```python
from build123d import *

# Parameters (mm, degrees)
F2_DEPTH = 3.2
F3_DEPTH = 3.15


with BuildPart() as f2:
    # F1 (on Front) → F2 (new body, symmetric)
    with BuildSketch(Plane.XZ):
        with BuildLine():
            Line((12, 6.3), (12, 0))
            Line((12, 0), (-12, 0))
            Line((-12, 0), (-12, 6.3))
            Line((-12, 6.3), (-15, 6.3))
            Line((-15, 6.3), (-15, 12.8))
            Line((-15, 12.8), (-20.6991873327, 12.8))
            ThreePointArc((-20.6991873327, 12.8), (-24.1218523847, 5.9585626477), (-25.3, -1.6))
            Line((-25.3, -1.6), (-25.3, -2.7))
            Line((-25.3, -2.7), (-23.56463857, -0.8764211088))
            Line((-23.56463857, -0.8764211088), (-21.7944681644, 7.4581257068))
            Line((-21.7944681644, 7.4581257068), (-18.7, 9.085327427))
            ThreePointArc((-18.7, 9.085327427), (-20.8621196327, 3.9359331242), (-21.6, -1.6))
            Line((-21.6, -1.6), (-21.6, -2.7))
            ThreePointArc((-21.6, -2.7), (-22.6837049096, -5.3162950904), (-25.3, -6.4))
            Line((-25.3, -6.4), (-29, -6.4))
            Line((-29, -6.4), (-29, -83.2))
            Line((-29, -83.2), (-21, -83.2))
            Line((-21, -83.2), (-21, -20))
            ThreePointArc((-21, -20), (-17.4852813742, -11.5147186258), (-9, -8))
            Line((-9, -8), (9, -8))
            ThreePointArc((9, -8), (17.4852813742, -11.5147186258), (21, -20))
            Line((21, -20), (21, -83.2))
            Line((21, -83.2), (29, -83.2))
            Line((29, -83.2), (29, -6.4))
            Line((29, -6.4), (25.3, -6.4))
            ThreePointArc((25.3, -6.4), (22.6837049096, -5.3162950904), (21.6, -2.7))
            Line((21.6, -2.7), (21.6, -1.6))
            ThreePointArc((21.6, -1.6), (20.8621196327, 3.9359331242), (18.7, 9.085327427))
            Line((18.7, 9.085327427), (21.7944681644, 7.4581257068))
            Line((21.7944681644, 7.4581257068), (23.56463857, -0.8764211088))
            Line((23.56463857, -0.8764211088), (25.3, -2.7))
            Line((25.3, -2.7), (25.3, -1.6))
            ThreePointArc((25.3, -1.6), (24.1218523847, 5.9585626477), (20.6991873327, 12.8))
            Line((20.6991873327, 12.8), (15, 12.8))
            Line((15, 12.8), (15, 6.3))
            Line((15, 6.3), (12, 6.3))
        make_face()
    extrude(amount=F2_DEPTH, both=True)

    # F1 (on Front) → F3 (join, symmetric)
    with BuildSketch(Plane.XZ):
        with BuildLine():
            Line((-20.6991873327, 12.8), (-15, 12.8))
            add(Edge.make_bspline(
                [(-14.9999999623, 12.8), (-13, 12.8), (-13.7499999859, 15.9999999397), (-14.4999999717, 19.1999998793), (-16.4999999623, 19.2)],
                knots=[6.0755071162, 6.0755071162, 6.0755071162, 7.6463034241, 7.6463034241, 9.217099732, 9.217099732, 9.217099732], degree=2, weights=[1, 0.7071067879, 1, 0.7071067879, 1]))
            Line((-16.5, 19.2), (-20, 19.2))
            ThreePointArc((-20, 19.2), (-26.653524819, 9.7318136236), (-29, -1.6))
            Line((-29, -1.6), (-29, -6.4))
            Line((-29, -6.4), (-25.3, -6.4))
            ThreePointArc((-25.3, -6.4), (-22.6837049096, -5.3162950904), (-21.6, -2.7))
            Line((-21.6, -2.7), (-21.6, -1.6))
            ThreePointArc((-21.6, -1.6), (-20.8621196327, 3.9359331242), (-18.7, 9.085327427))
            Line((-18.7, 9.085327427), (-21.7944681644, 7.4581257068))
            Line((-21.7944681644, 7.4581257068), (-23.56463857, -0.8764211088))
            Line((-23.56463857, -0.8764211088), (-25.3, -2.7))
            Line((-25.3, -2.7), (-25.3, -1.6))
            ThreePointArc((-25.3, -1.6), (-24.1218523847, 5.9585626477), (-20.6991873327, 12.8))
        make_face()
        with BuildLine():
            add(Edge.make_bspline(
                [(16.5, 19.2), (14.5000000377, 19.2), (13.7500000377, 16), (13.0000000377, 12.8), (15, 12.8)],
                knots=[0.2076781757, 0.2076781757, 0.2076781757, 1.7784745025, 1.7784745025, 3.3492708293, 3.3492708293, 3.3492708293], degree=2, weights=[1, 0.7071067812, 1, 0.7071067812, 1]))
            Line((15, 12.8), (20.6991873327, 12.8))
            ThreePointArc((20.6991873327, 12.8), (24.1218523847, 5.9585626477), (25.3, -1.6))
            Line((25.3, -1.6), (25.3, -2.7))
            Line((25.3, -2.7), (23.56463857, -0.8764211088))
            Line((23.56463857, -0.8764211088), (21.7944681644, 7.4581257068))
            Line((21.7944681644, 7.4581257068), (18.7, 9.085327427))
            ThreePointArc((18.7, 9.085327427), (20.8621196327, 3.9359331242), (21.6, -1.6))
            Line((21.6, -1.6), (21.6, -2.7))
            ThreePointArc((21.6, -2.7), (22.6837049096, -5.3162950904), (25.3, -6.4))
            Line((25.3, -6.4), (29, -6.4))
            Line((29, -6.4), (29, -1.6))
            ThreePointArc((29, -1.6), (26.653524819, 9.7318136236), (20, 19.2))
            Line((20, 19.2), (16.5, 19.2))
        make_face()
    extrude(amount=F3_DEPTH, both=True)


solid = f2.part
```
CAD build for the part. Positions are in the model's coordinates, mm. A direction names the side the tool comes from. Give positions to 0.01 mm unless a question says otherwise; leave off trailing zeros. Order: outer loops, then holes, each group sorted by start corner. A loop starts at its lowest first (then second) coordinate and runs counter-clockwise, first axis right, second up.
(1) Mould opens along X. For faces 1 (the flat face through (21, 0, -51)), 2 (the flat face through (29, 0, -43)), 3 (the cylindrical face through (17.39, -0.04, -11.42)), 4 (the flat face through (-18, 0, 19.2)) say: released by +X, released by -X, zero draft, split by the parting line, or undercut.
(2) Flat gauge pins, fed straight in: pin 1 (3 mm diameter, centred on x = -9, y = 2, fed in from +Z); pin 2 (3 mm diameter, centred on x = 17.5, y = -0.5, fed in from -Z); pin 3 (1.5 mm diameter, centred on x = 13.5, y = 0, fed in from +Z). Where does each tip first touch, or does it go through?
(3) Tool access for faces 5 (the flat face through (-22, -3.2, -31)), 6 (the flat face through (0, 0, 0)), 7 (the flat face through (-21, 0, -52)): list every direction of +Z, -Z, +X, -X, +Y, -Y with a clear straight run to the whole face (end or side of a thin tool).
(4) Drill centre lines: L1, parallel to X at y = 3, z = -29.5; L2, parallel to Z at x = -6.5, y = -3; L3, parallel to Y at x = 25.5, z = 10. Where is each one in solid material? Low to high.
(5) Saw through at B-B, the plane z = 10.5. Give the cut face in (x, y).
(6) Saw through at C-C, the plane x = 11. Give the cut face in (y, z).
(7) Saw through at A-A, the plane z = -42. Give the cut face in (x, y).
Results found:
1. face 1: undercut
1. face 2: released by +X
1. face 3: undercut
1. face 4: zero draft
2. pin 1: stops at z = 0
2. pin 2: stops at z = -13.37
2. pin 3: stops at z = 17.34
3. face 5: +Z, -Z, +X, -X, -Y
3. face 6: +Z, +Y, -Y
3. face 7: -Z, +Y, -Y
4. L1: x = -29 to -21, 21 to 29
4. L2: z = -8 to 0
4. L3: y = -3.15 to 3.15
5. outline: (-26.31, -3.15) - (-22.15, -3.15) - (-22.15, -3.2) - (-15, -3.2) - (-15, 3.2) - (-22.15, 3.2) - (-22.15, 3.15) - (-26.31, 3.15) - close; (15, -3.2) - (22.15, -3.2) - (22.15, -3.15) - (26.31, -3.15) - (26.31, 3.15) - (22.15, 3.15) - (22.15, 3.2) - (15, 3.2) - close
6. outline: (-3.2, -8.17) - (3.2, -8.17) - (3.2, 0) - (-3.2, 0) - close
7. outline: (-29, -3.2) - (-21, -3.2) - (-21, 3.2) - (-29, 3.2) - close; (21, -3.2) - (29, -3.2) - (29, 3.2) - (21, 3.2) - close
